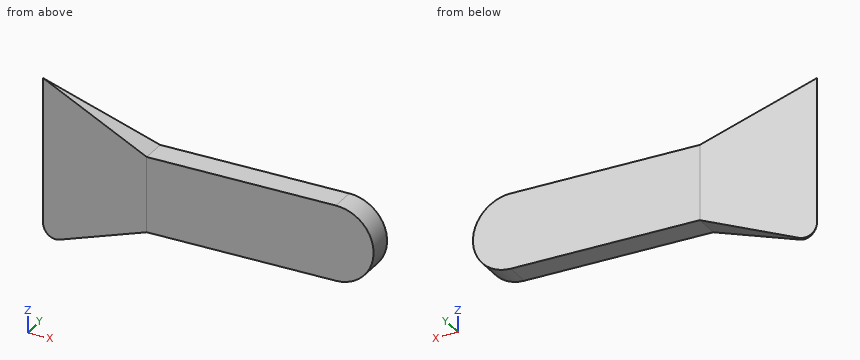
from build123d import *

# Parameters (mm, degrees)
BOSS_EXTRUDE1_DEPTH     = 2
CUT_EXTRUDE1_DEPTH      = 22.314348222
CUT_EXTRUDE1_DEPTH_BACK = 22.314348222
CUT_EXTRUDE2_DEPTH      = 22.314348222
CUT_EXTRUDE2_DEPTH_BACK = 22.314348222


with BuildPart() as part:
    # Sketch1 → Boss-Extrude1 (new body)
    with BuildSketch(Plane(origin=(0, 0, 0), x_dir=(1, 0, 0), z_dir=(0, 1, 0))):
        with BuildLine():
            Line((2.182949987, 3), (-5.217733039, 5.909415386))
            ThreePointArc((-5.217733039, 5.909415386), (-6.146688679, 5.80514872), (-6.583603739, 4.978749694))
            Line((-6.583603739, 4.978749694), (-6.583603739, -6.553622658))
            Line((-6.583603739, -6.553622658), (2.182949987, -3))
            Line((2.182949987, -3), (17.182949987, -3))
            ThreePointArc((17.182949987, -3), (20.182949987, 0), (17.182949987, 3))
            Line((17.182949987, 3), (2.182949987, 3))
        make_face()
    extrude(amount=BOSS_EXTRUDE1_DEPTH)

    # Sketch2 → Cut-Extrude1 (cut, two sides: drawn at the far end of the back side and taken through both)
    with BuildSketch(Plane.XY.offset(-CUT_EXTRUDE1_DEPTH_BACK)):
        Polygon((-6.583603739, 1), (2.182949987, 2), (-6.583603739, 2), align=None)
    extrude(amount=CUT_EXTRUDE1_DEPTH + CUT_EXTRUDE1_DEPTH_BACK, mode=Mode.SUBTRACT)

    # Sketch3 → Cut-Extrude2 (cut, two sides: drawn at the far end of the back side and taken through both)
    with BuildSketch(Plane.XY.offset(-CUT_EXTRUDE2_DEPTH_BACK)):
        Polygon((-6.583603739, 1), (-6.583603739, 0), (2.182949987, 0), align=None)
    extrude(amount=CUT_EXTRUDE2_DEPTH + CUT_EXTRUDE2_DEPTH_BACK, mode=Mode.SUBTRACT)


solid = part.part
Verification items for the finished model (mm, model axes). Give positions to 0.01 mm unless a question says otherwise; leave off trailing zeros. Loops run counter-clockwise (first coordinate to the right, second up) from the corner with the lowest first, then second, coordinate; pieces in that order, holes last.
1) Depth check by flat-ended pin: pin 1 Ø1 at (x, y) = (12, 1) entering from -Z; pin 2 Ø1 at (x, z) = (-2.5, -1) entering from -Y. Enter the tip coordinate at first touch or a pass-through.
2) Sectioned sample at C-C, the plane y = 1.5. Enter the section's corners in (x, z).
3) Sectioned sample at A-A, the plane z = 0. Enter the section's corners in (x, y), then the cut area to 3 significant figures.
4) Sectioned sample at B-B, the plane x = 9.5. Enter the section's corners in (y, z).
5) Sectioned sample at D-D, the plane z = -2.75. Enter the section's corners in (x, y), then the cut area to 3 significant figures.
6) Thickness scan on line 1 along Z through (x, y) = (9.25, 1.85); line 2 along Z through (x, y) = (-4, 0.8); line 3 along Y through (x, z) = (-2.5, -2.75). Record the ranges inside material, lowest first.
Answers:
1. pin 1: stops at z = -3
1. pin 2: stops at y = 0.48
2. outline: (-2.2, -4.72) - (2.18, -3) - (17.18, -3) arc R3 ccw to (17.18, 3) - (2.18, 3) - (-2.2, 4.78) - close
3. outline: (-6.58, 1) - (2.18, 0) - (20.18, 0) - (20.18, 2) - (2.18, 2) - close
3. area: 44.8 mm2
4. outline: (0, -3) - (2, -3) - (2, 3) - (0, 3) - close
5. outline: (-6.58, 1) - (2.18, 0) - (18.38, 0) - (18.38, 2) - (2.18, 2) - close
5. area: 41.2 mm2
6. line 1: z = -3 to 3
6. line 2: z = -5.43 to 5.51
6. line 3: y = 0.53 to 1.47
